Geometry check sheet. Reference: the model listing, model coordinates, mm. A direction names the side the tool comes from. Round coordinates to 2 decimals unless told otherwise and drop trailing zeros. Order: outer loops, then holes, each group sorted by start corner. A loop starts at its lowest first (then second) coordinate and runs counter-clockwise, first axis right, second up.
```python
from build123d import *

# Parameters (mm, degrees)
F2_DEPTH = 3.6
F4_DEPTH = 3.6
F5_W     = 40.3048
F5_H     = 1.8
F6_DEPTH = 1.8
F7_R     = 1.9
F8_R     = 0.5


with BuildPart() as f2:
    # F1 (on Top) → F2 (new body)
    with BuildSketch(Plane.XY):
        with BuildLine():
            Line((-20.1524, -54.15), (20.1524, -54.15))
            ThreePointArc((20.1524, -54.15), (24.3933436308, -52.3933436308), (26.15, -48.1524))
            Line((26.15, -48.1524), (26.15, 48.1524))
            ThreePointArc((26.15, 48.1524), (24.3933436308, 52.3933436308), (20.1524, 54.15))
            Line((20.1524, 54.15), (-20.1524, 54.15))
            ThreePointArc((-20.1524, 54.15), (-24.3933436308, 52.3933436308), (-26.15, 48.1524))
            Line((-26.15, 48.1524), (-26.15, -48.1524))
            ThreePointArc((-26.15, -48.1524), (-24.3933436308, -52.3933436308), (-20.1524, -54.15))
        make_face()
    extrude(amount=F2_DEPTH)

    # F3 (on face) → F4 (join)
    with BuildSketch(Plane.XZ.offset(54.15)):
        Polygon((9, 3.6), (-9, 3.6), (-9, 1.8), (-9, 0), (9, 0), (9, 1.8), align=None)
    extrude(amount=F4_DEPTH)

    # F5 (on face) → F6 (join)
    with BuildSketch(Plane(origin=(0, 54.15, 0), x_dir=(-1, 0, 0), z_dir=(0, 1, 0))):
        with Locations((0, 0.9)):
            Rectangle(F5_W, F5_H)
    extrude(amount=F6_DEPTH)

    # F7
    f7_edges = [f2.edges().sort_by_distance(p)[0] for p in [
        (0, -57.75, 3.6),
    ]]
    fillet(f7_edges, radius=F7_R)

    # F8
    f8_edges = [f2.edges().sort_by_distance(p)[0] for p in [
        (0, 55.95, 1.8),
    ]]
    fillet(f8_edges, radius=F8_R)


solid = f2.part
```
(1) Depth check by flat-ended pin: P1, Ø0.6, axis at x = 2.5, y = 55, coming from the +Z side; P2, Ø1.4, axis at y = 55, z = 1.5, coming from the +X side; P3, Ø2, axis at x = 17, y = -44, coming from the -Z side; P4, Ø1.8, axis at y = -56, z = 2.5, coming from the +X side. Enter the tip coordinate at first touch or a pass-through.
Returned:
P1: stops at z = 1.8
P2: stops at x = 20.15
P3: stops at z = 0
P4: stops at x = 9
(2) Sectioned sample at B-B, the plane x = 15. Record the cut outline in (y, z).
Returned:
outline: (-54.15, 0) - (55.95, 0) - (55.95, 1.3) arc R0.5 ccw to (55.45, 1.8) - (54.15, 1.8) - (54.15, 3.6) - (-54.15, 3.6) - close
(3) Set-up check for faces 1 (the flat face through (14, -54.15, 2)), 2 (the flat face through (-9, -56, 2)), 3 (the flat face through (0, -2, 0)): record each of +Z, -Z, +X, -X, +Y, -Y from which the full face is reachable in a straight line by a thin tool's end or side.
Returned:
face 1: +Z, -Z, +X, -Y
face 2: +Z, -Z, -X, -Y
face 3: -Z, +X, -X, +Y, -Y
(4) Sectioned sample at A-A, the plane z = 0.6. Record the cut outline in (x, y), and give its area (3 significant figures).
Returned:
outline: (-26.15, -48.15) arc R6 ccw to (-20.15, -54.15) - (-9, -54.15) - (-9, -57.75) - (9, -57.75) - (9, -54.15) - (20.15, -54.15) arc R6 ccw to (26.15, -48.15) - (26.15, 48.15) arc R6 ccw to (20.15, 54.15) - (20.15, 55.95) - (-20.15, 55.95) - (-20.15, 54.15) arc R6 ccw to (-26.15, 48.15) - close
area: 5,770 mm2
(5) Material ranges on line 1 (Y direction, x = 18, z = 0.8); line 2 (Y direction, x = -11.5, z = 3.1); line 3 (X direction, y = -51, z = 2.3), recorded low to high.
Returned:
line 1: y = -54.15 to 55.95
line 2: y = -54.15 to 54.15
line 3: x = -25.43 to 25.43
(6) Sectioned sample at C-C, the plane x = 22. Record the cut outline in (y, z), and give its area (3 significant figures).
Returned:
outline: (-53.86, 0) - (53.86, 0) - (53.86, 3.6) - (-53.86, 3.6) - close
area: 388 mm2
